from build123d import *

# Parameters (mm, degrees)
F0_W      = 60
F0_H      = 100
F0_W_2    = 45
F0_H_2    = 40
F1_DEPTH  = 4
F3_D      = 3.5
F3_DEPTH  = 25
F3_TIP    = 1.0515060833
F5_R      = 5
F6_R      = 2
F8_D      = 3.5
F8_DEPTH  = 25
F8_TIP    = 1.0515060833
F4_R      = 3.75
F4_R_2    = 1.6
F9_DEPTH  = 25
F10_DEPTH = 25


# Not quite as in the source:
# - a feature names something its author has since deleted; it is built from what else it names


with BuildPart() as f1:
    # F0 (on Front) → F1 (new body)
    with BuildSketch(Plane.XZ):
        Rectangle(F0_W, F0_H)
        with Locations((0, 22)):
            Rectangle(F0_W_2, F0_H_2, mode=Mode.SUBTRACT)
    extrude(amount=F1_DEPTH)

    # F3
    with Locations(Plane.XZ.offset(4)):
        with Locations((-26, 46), (26, 46), (26, -46), (-26, -46)):
            Hole(F3_D / 2, depth=F3_DEPTH)
            with Locations((0, 0, -(F3_DEPTH + F3_TIP / 2))):  # 118° drill point
                Cone(0, F3_D / 2, F3_TIP, mode=Mode.SUBTRACT)

    # F5
    f5_edges = [f1.edges().sort_by_distance(p)[0] for p in [
        (-30, -2, 50),
        (-30, -2, -50),
        (30, -2, -50),
        (30, -2, 50),
    ]]
    fillet(f5_edges, radius=F5_R)

    # F6
    f6_edges = [f1.edges().sort_by_distance(p)[0] for p in [
        (-22.5, -2, 2),
        (-22.5, -2, 42),
        (22.5, -2, 42),
        (22.5, -2, 2),
    ]]
    fillet(f6_edges, radius=F6_R)

    # F8
    with Locations(Plane.XZ.offset(4)):
        with Locations((-25, -2), (25, -2)):
            Hole(F8_D / 2, depth=F8_DEPTH)
            with Locations((0, 0, -(F8_DEPTH + F8_TIP / 2))):  # 118° drill point
                Cone(0, F8_D / 2, F8_TIP, mode=Mode.SUBTRACT)

    # F4 (on face) → F9 (cut)
    with BuildSketch(Plane.XZ.offset(4)):
        with Locations((0, -25)):
            Circle(F4_R)
        with Locations((-7.8, -25)):
            Circle(F4_R_2)
    extrude(amount=-F9_DEPTH, mode=Mode.SUBTRACT)

    # F4 (on face) → F10 (cut)
    with BuildSketch(Plane.XZ.offset(4)):
        with Locations((0, -25)):
            Circle(F4_R)
        with Locations((-7.8, -25)):
            Circle(F4_R_2)
    extrude(amount=-F10_DEPTH, mode=Mode.SUBTRACT)


solid = f1.part
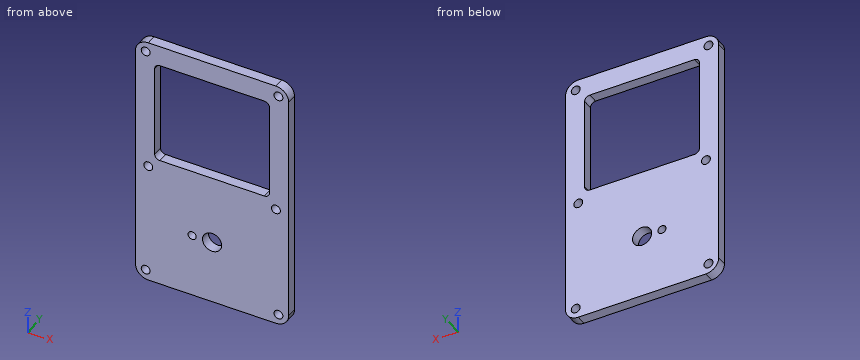
Could you check a few things on this model? Use its own coordinates, in mm. Give positions to 0.01 mm unless a question says otherwise; leave off trailing zeros. Order: outer loops, then holes, each group sorted by start corner. A loop starts at its lowest first (then second) coordinate and runs counter-clockwise, first axis right, second up. Notation, with made-up numbers: (-17, 52) - (29, 52) arc R31 ccw to (29, 76) - close; hole circle Ø1 at (-26, -19.75). An arc over 180 degrees is marked (long way). Return JSON: item names as keys, results as strings. Group by question number.
Q1. Suppose I cut it at D-D, the plane x = -7.8. Please give me the cut outline in (y, z).
Q2. Suppose I cut it at B-B, the plane x = -19. Please give me the cut outline in (y, z), and give its area (3 significant figures).
Q3. Will this pin go through, and if not, where does the flat tip stop? pin 1 Ø3 at (x, z) = (-26, -46) entering from +Y.
Q4. Please list where these lines run through material, in increasing order: line 1 along Z through (x, y) = (0, -2.25); line 2 along Z through (x, y) = (-7.8, -2.8); line 3 along X through (y, z) = (-0.3, 36.5). Write a range as [from, to].
Q5. Suppose I cut it at C-C, the plane z = 39. Please give me the cut outline in (x, y).
Q6. Suppose I cut it at A-A, the plane z = -2. Please give me the cut outline in (x, y), and give its area (3 significant figures).
Resolved:
{
 "1": {"outline": "(-4, -50) - (0, -50) - (0, -26.6) - (-4, -26.6) - close; (-4, -23.4) - (0, -23.4) - (0, 2) - (-4, 2) - close; (-4, 42) - (0, 42) - (0, 50) - (-4, 50) - close"},
 "2": {"outline": "(-4, -50) - (0, -50) - (0, 2) - (-4, 2) - close; (-4, 42) - (0, 42) - (0, 50) - (-4, 50) - close", "area": "240 mm2"},
 "3": {"pin 1": "passes through"},
 "4": {"line 1": "z = [-50, -28.75], [-21.25, 2], [42, 50]", "line 2": "z = [-50, -26.6], [-23.4, 2], [42, 50]", "line 3": "x = [-30, -22.5], [22.5, 30]"},
 "5": {"outline": "(-30, -4) - (-22.5, -4) - (-22.5, 0) - (-30, 0) - close; (22.5, -4) - (30, -4) - (30, 0) - (22.5, 0) - close"},
 "6": {"outline": "(-30, -4) - (-26.75, -4) - (-26.75, 0) - (-30, 0) - close; (-23.25, -4) - (23.25, -4) - (23.25, 0) - (-23.25, 0) - close; (26.75, -4) - (30, -4) - (30, 0) - (26.75, 0) - close", "area": "212 mm2"}
}
